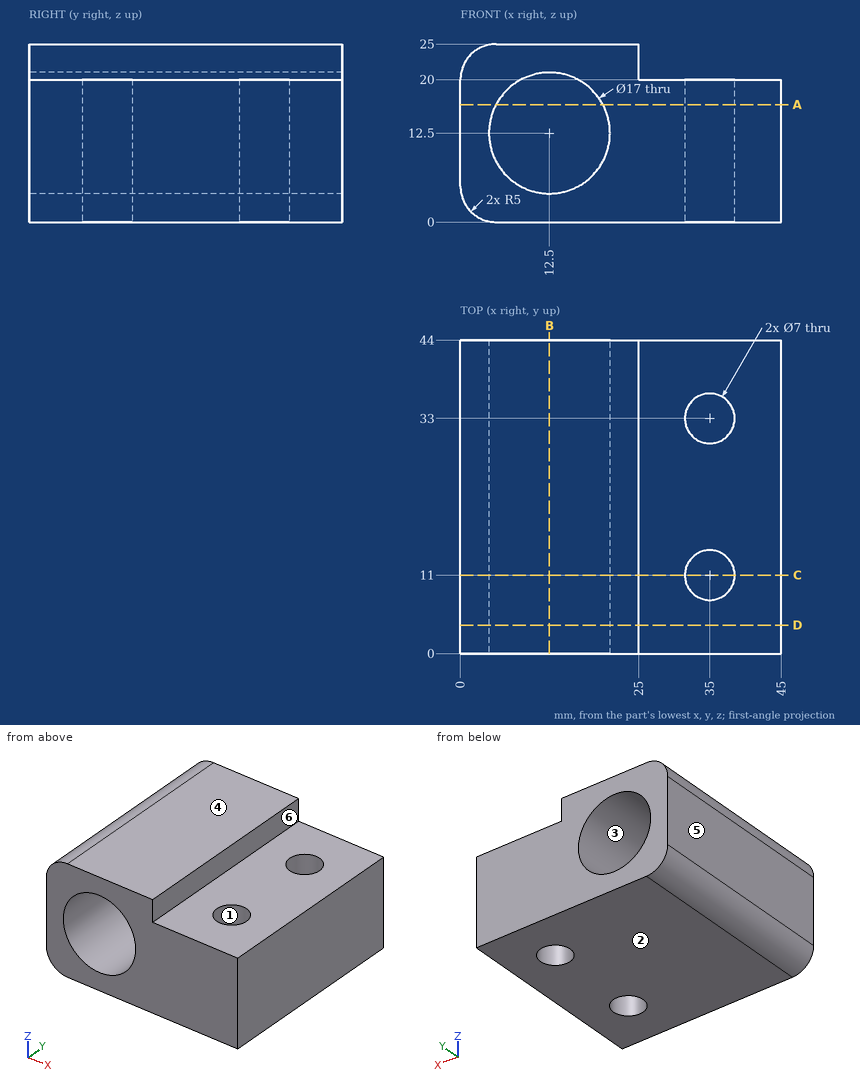
Job drawing, mm, ordinate dimensions from the low corner. One solid piece. A direction names the side the tool comes from. Give positions to 0.01 mm unless a question says otherwise; leave off trailing zeros. Loops run counter-clockwise (first coordinate to the right, second up) from the corner with the lowest first, then second, coordinate; pieces in that order, holes last.
Item 1: Drill centre lines: line 1 (Y direction, x = 35, z = 15.25); line 2 (X direction, y = 11.5, z = 8.5); line 3 (Z direction, x = 26, y = 24). Where is each one in solid material? Low to high.
Answers follow:
line 1: y = 0 to 7.5, 14.5 to 29.5, 36.5 to 44
line 2: x = 0 to 5, 20 to 31.54, 38.46 to 45
line 3: z = 0 to 20
Item 2: Slice it at C-C, the plane y = 11. List the corners of the cut face in (x, z).
Answers follow:
outline: (0, 5) arc R5 ccw to (5, 0) - (31.5, 0) - (31.5, 20) - (25, 20) - (25, 25) - (5, 25) arc R5 ccw to (0, 20) - close; (38.5, 0) - (45, 0) - (45, 20) - (38.5, 20) - close; hole circle Ø17 at (12.5, 12.5)
Item 3: Pull direction Z, two halves, no side cores. Call the marked faces 1, 2, 3 and 4: released by +Z, released by -Z, zero draft, split by the parting line, or undercut.
Answers follow:
face 1: zero draft
face 2: released by -Z
face 3: undercut
face 4: released by +Z
Item 4: Slice it at B-B, the plane x = 12.5. List the corners of the cut face in (y, z).
Answers follow:
outline: (0, 0) - (44, 0) - (44, 4) - (0, 4) - close; (0, 21) - (44, 21) - (44, 25) - (0, 25) - close
Item 5: Slice it at A-A, the plane z = 16.5. List the corners of the cut face in (x, y), and give its area (3 significant figures).
Answers follow:
outline: (0, 0) - (5, 0) - (5, 44) - (0, 44) - close; (20, 0) - (45, 0) - (45, 44) - (20, 44) - close; hole circle Ø7 at (35, 11); hole circle Ø7 at (35, 33)
area: 1,240 mm2
Item 6: Which spindle directions (+Z, -Z, +X, -X, +Y, -Y) get a long thin tool onto all of the face, cutting with end or side? Do the marked faces 5 and 6. Say none if no direction does.
Answers follow:
face 5: +Z, -Z, -X, +Y, -Y
face 6: +Z, +X, +Y, -Y
Item 7: Slice it at D-D, the plane y = 4. List the corners of the cut face in (x, z), and give its area (3 significant figures).
Answers follow:
outline: (0, 5) arc R5 ccw to (5, 0) - (45, 0) - (45, 20) - (25, 20) - (25, 25) - (5, 25) arc R5 ccw to (0, 20) - close; hole circle Ø17 at (12.5, 12.5)
area: 787 mm2
Item 8: Flat gauge pins, fed straight in: pin 1 (2 mm diameter, centred on x = 14.5, z = 18, fed in from +Y); pin 2 (1.5 mm diameter, centred on x = 33.5, z = 20.5, fed in from +Y); pin 3 (4 mm diameter, centred on y = 13.5, z = 22.5, fed in from +X). Where does each tip first touch, or does it go through?
Answers follow:
pin 1: passes through
pin 2: stops at y = 44
pin 3: stops at x = 25
